Autodesk Inventor part; units mm, degrees
ref_plane "Work Plane1" through (0, 0, -15.24) normal (0, 0, -1) x (-1, 0, 0)
ref_plane "YZ Plane" through (0, 0, 0) normal (1, 0, 0) x (0, 1, 0)
ref_plane "XZ Plane" through (0, 0, 0) normal (0, 1, 0) x (-1, 0, 0)
sketch "Sketch1" plane through (0, 0, 0) normal (0, 0, 1) x (1, 0, 0)
  line L0 (-6.5322, -3.0499) -> (-5.8184, 4.2476)
  line L1 (-5.8184, 4.2476) -> (0.8584, 7.2782)
  line L2 (0.8584, 7.2782) -> (6.8213, 3.0112)
  line L3 (6.8213, 3.0112) -> (6.1075, -4.2863)
  line L4 (6.1075, -4.2863) -> (-0.5693, -7.3169)
  line L5 (-0.5693, -7.3169) -> (-6.5322, -3.0499)
  circle A0 centre (0.1445, -0.0193) radius 15.5
  line L6 (-6.7574, 4.9196) -> (-7.5837, -3.5272)
  line L7 (-7.5837, -3.5272) -> (-0.6817, -8.4661)
  line L8 (-0.6817, -8.4661) -> (7.0465, -4.9582)
  line L9 (7.0465, -4.9582) -> (7.8727, 3.4885)
  line L10 (7.8727, 3.4885) -> (0.9708, 8.4274)
  line L11 (0.9708, 8.4274) -> (-6.7574, 4.9196)
  circle A1 centre (0.1445, -0.0193) radius 8.487
  point P0 (0, 0)
  dimension "d0" = 1
extrude "Extrusion1" add sketch "Sketch1" along normal blind 1.5 contours L0 L1 L2 L3 L4 L5 | L11 L10 L9 L8 L7 L6 | A1 L11 | L6 A1 | L7 A1 | A1 L10 | L8 A1 | A1 L9
sketch "Sketch2" plane through (0, 0, 0) normal (0, 0, -1) x (-1, 0, 0)
  line L0 (5.8184, 4.2476) -> (6.5322, -3.0499)
  line L1 (6.5322, -3.0499) -> (0.5693, -7.3169)
  line L2 (0.5693, -7.3169) -> (-6.1075, -4.2863)
  line L3 (-6.1075, -4.2863) -> (-6.8213, 3.0112)
  line L4 (-6.8213, 3.0112) -> (-0.8584, 7.2782)
  line L5 (-0.8584, 7.2782) -> (5.8184, 4.2476)
  circle A0 centre (-0.1445, -0.0193) radius 15.5
  line L6 (5.8184, 4.2476) -> (6.5322, -3.0499)
  line L7 (6.5322, -3.0499) -> (0.5693, -7.3169)
  line L8 (0.5693, -7.3169) -> (-6.1075, -4.2863)
  line L9 (-6.1075, -4.2863) -> (-6.8213, 3.0112)
  line L10 (-6.8213, 3.0112) -> (-0.8584, 7.2782)
  line L11 (-0.8584, 7.2782) -> (5.8184, 4.2476)
  circle A1 centre (-0.1445, -0.0193) radius 15.5
  point P0 (0, 0)
extrude "Extrusion2" add sketch "Sketch2" along normal blind 18.24 contours L0 L1 L2 L3 L4 L5
ref_plane "Work Plane1" through (0, 0, -15.24) normal (0, 0, -1) x (-1, 0, 0)
sketch "Sketch3" plane through (0, 0, -15.24) normal (0, 0, -1) x (-1, 0, 0)
  line L0 (5.8184, 4.2476) -> (6.5322, -3.0499)
  line L1 (-0.8584, 7.2782) -> (5.8184, 4.2476)
  line L2 (-6.8213, 3.0112) -> (-0.8584, 7.2782)
  line L3 (-6.1075, -4.2863) -> (-6.8213, 3.0112)
  line L4 (0.5693, -7.3169) -> (-6.1075, -4.2863)
  line L5 (6.5322, -3.0499) -> (0.5693, -7.3169)
  circle A0 centre (0, 0) radius 4.9486
  dimension "d17" = 9.8971
sketch "Sketch4" plane through (0, 0, 1.5) normal (0, 0, 1) x (1, 0, 0)
  circle A0 centre (0, 0) radius 3
  dimension "d8" = 6
extrude "Extrusion4" cut sketch "Sketch4" against normal through all
extrude "Extrusion6" cut sketch "Sketch3" along normal blind 1.5
sketch "Sketch6" plane through (0, 0, -18.24) normal (0, 0, -1) x (-1, 0, 0)
  circle A0 centre (0, 0) radius 3
  line L0 (5.8184, 4.2476) -> (6.5322, -3.0499)
  line L1 (-0.8584, 7.2782) -> (5.8184, 4.2476)
  line L2 (-6.8213, 3.0112) -> (-0.8584, 7.2782)
  line L3 (-6.1075, -4.2863) -> (-6.8213, 3.0112)
  line L4 (0.5693, -7.3169) -> (-6.1075, -4.2863)
  line L5 (6.5322, -3.0499) -> (0.5693, -7.3169)
  circle A1 centre (0, 0) radius 6.2043
extrude "Extrusion7" cut sketch "Sketch6" against normal up to surface (1.5 mm away)
properties part number "Hub"
The model under review builds one solid part; all positions refer to its coordinate system, in mm. A direction names the side the tool comes from. Coordinates: 2 decimals unless noted, no trailing zeros. Order: outer loops, then holes, each group sorted by start corner. A loop starts at its lowest first (then second) coordinate and runs counter-clockwise, first axis right, second up. Notation, with made-up numbers: (88, 8) -> (102, 8) arc R4 cw to (102, 14) -> close; hole circle Ø10 at (-28, 70.25). An arc over 180 degrees is marked (long way). Answer in a Markdown table with one row per item.
(1) Consider section D-D (x = 0). Write out the cut boundary in (y, z).
Answers:
| item | result |
|---|---|
| outline | (-8.51, 0) -> (-7.06, 0) -> (-7.06, -15.24) -> (-4.95, -15.24) -> (-4.95, -16.74) -> (-6.2, -16.74) -> (-6.2, -18.24) -> (-3, -18.24) -> (-3, 1.5) -> (-8.51, 1.5) -> close; (3, -18.24) -> (6.2, -18.24) -> (6.2, -16.74) -> (4.95, -16.74) -> (4.95, -15.24) -> (6.89, -15.24) -> (6.89, 0) -> (8.47, 0) -> (8.47, 1.5) -> (3, 1.5) -> close |
(2) Consider section A-A (z = -9.75). Write out the cut boundary in (x, y), plus the area to 3 significant figures.
Answers:
| item | result |
|---|---|
| outline | (-6.53, -3.05) -> (-0.57, -7.32) -> (6.11, -4.29) -> (6.82, 3.01) -> (0.86, 7.28) -> (-5.82, 4.25) -> close; hole circle Ø6 at (0, 0) |
| area | 111 mm² |
(3) The part is to be moulded in two halves that separate along Z. For faces 1 (the flat face through (-3, 6, 0)), 2 (the cylindrical face through (-6.59, 5.145, 0.74)), 3 (the cylindrical face through (1.07, 4.83, -15.98)), say which applies: +Z half, -Z half, draft (parallel to the pull), parting line (faces both ways), or undercut.
Answers:
| item | result |
|---|---|
| face 1 | -Z half |
| face 2 | draft |
| face 3 | undercut |
(4) Wall thickness on line 1 along Z through (x, y) = (-2, 5); line 2 along Z through (x, y) = (6, -2.5); line 3 along Y through (x, z) = (0.5, -14.25): over which ranges is each line inside the solid? List them lowest first.
Answers:
| item | result |
|---|---|
| line 1 | -18.24 to -16.74, -15.24 to 1.5 |
| line 2 | -15.24 to 1.5 |
| line 3 | -6.83 to -2.96, 2.96 to 7.12 |
(5) Consider section B-B (x = 5.75). Write out the cut boundary in (y, z).
Answers:
| item | result |
|---|---|
| outline | (-6.39, 0) -> (-4.45, 0) -> (-4.45, -15.24) -> (3.78, -15.24) -> (3.78, 0) -> (6.35, 0) -> (6.35, 1.5) -> (-6.39, 1.5) -> close; (-2.33, -18.24) -> (2.33, -18.24) -> (2.33, -16.74) -> (-2.33, -16.74) -> close |
(6) Consider section C-C (y = 5.25). Write out the cut boundary in (x, z), plus the area to 3 significant figures.
Answers:
| item | result |
|---|---|
| outline | (-6.51, 0) -> (-3.61, 0) -> (-3.61, -15.24) -> (3.69, -15.24) -> (3.69, 0) -> (6.8, 0) -> (6.8, 1.5) -> (-6.51, 1.5) -> close; (-3.31, -18.24) -> (3.31, -18.24) -> (3.31, -16.74) -> (-3.31, -16.74) -> close |
| area | 141 mm² |
(7) Insertion check: pin 1 (5 mm diameter, centred on x = 2, z = -4.5, fed in from +Y); pin 2 (1.5 mm diameter, centred on y = 4.5, z = -9, fed in from +X); pin 3 (2 mm diameter, centred on y = -3, z = -6.5, fed in from -X); pin 4 (6 mm diameter, centred on x = 2, y = 0.5, fed in from +Z). Each pin has a flat end and moves straight along its axis. Give the tip position at first contact, or say it passes through.
Answers:
| item | result |
|---|---|
| pin 1 | y = 7.28 |
| pin 2 | x = 5.79 |
| pin 3 | x = -6.53 |
| pin 4 | z = 1.5 |
(8) Machinability: for faces 4 (the flat face through (5, -1, -15.24)), 5 (the flat face through (-6.17, 0.65, -7.51)), 6 (the flat face through (6.46, -0.69, -7.51)), which of the approach directions +Z, -Z, +X, -X, +Y, -Y give a long, thin tool a straight path to every point of the face, cutting with its end or side? Answer none if there is none.
Answers:
| item | result |
|---|---|
| face 4 | none |
| face 5 | -Z, -X, +Y |
| face 6 | -Z, +X, -Y |
